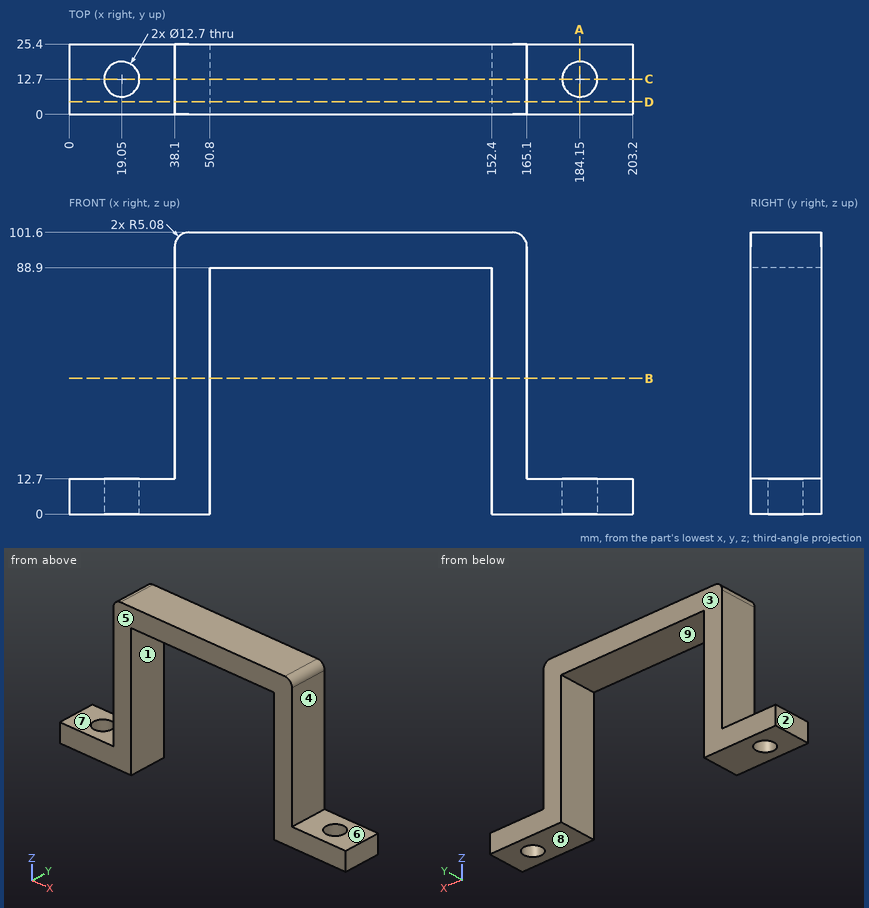
Geometry: see drawing. Coordinates: mm, zero at the bounding-box minimum. A direction names the side the tool comes from. Coordinates: 2 decimals unless noted, no trailing zeros. Order: outer loops, then holes, each group sorted by start corner. A loop starts at its lowest first (then second) coordinate and runs counter-clockwise, first axis right, second up. Notation, with made-up numbers: (-27.5, 40) -> (14.5, 40) arc R10 cw to (14.5, 55) -> close; hole circle Ø9 at (81.25, -12.75). An arc over 180 degrees is marked (long way). Write each question's results on one line, items separated by ' | '. Start each with the question number.
1) Cut plane A-A, the plane x = 184.15. Output: boundary loops of the cut face in (y, z), and give its area (3 significant figures).
2) Material intervals for line 1 along X through (y, z) = (8, 68); line 2 along Y through (x, z) = (19, 5); line 3 along Z through (x, y) = (85.5, 11.25), sorted ascending.
3) Cut plane B-B, the plane z = 49. Output: boundary loops of the cut face in (x, y).
4) Cut plane C-C, the plane y = 12.7. Output: boundary loops of the cut face in (x, z), and give its area (3 significant figures).
5) Set-up query: the marked faces 5, 6, 7, 8 and 9. Return all of +Z, -Z, +X, -X, +Y, -Y with unobstructed straight access to the full face (end or side cutting, diameter ignored); none if empty.
6) Cut plane D-D, the plane y = 4.5. Output: boundary loops of the cut face in (x, z).
7) Mould query, pull axis X, two halves, no side actions, for the marked faces 1, 2, 3 and 4. Classes: released by +X, released by -X, zero draft, split by the parting line, or undercut.
8) First-contact query: pin 1 (14.5 mm diameter, centred on x = 184.15, y = 12.7, fed in from +Z); pin 2 (5 mm diameter, centred on x = 142, y = 4.5, fed in from -Z); pin 3 (2 mm diameter, centred on y = 18.5, z = 77.5, fed in from +X). Flat tips, straight axial feed; report the tip coordinate or a pass-through.
Checks:
1) outline: (0, 0) -> (6.35, 0) -> (6.35, 12.7) -> (0, 12.7) -> close; (19.05, 0) -> (25.4, 0) -> (25.4, 12.7) -> (19.05, 12.7) -> close | area: 161 mm^2
2) line 1: 38.1 to 50.8, 152.4 to 165.1 | line 2: 0 to 6.35, 19.05 to 25.4 | line 3: 88.9 to 101.6
3) outline: (38.1, 0) -> (50.8, 0) -> (50.8, 25.4) -> (38.1, 25.4) -> close; (152.4, 0) -> (165.1, 0) -> (165.1, 25.4) -> (152.4, 25.4) -> close
4) outline: (0, 0) -> (12.7, 0) -> (12.7, 12.7) -> (0, 12.7) -> close; (25.4, 0) -> (50.8, 0) -> (50.8, 88.9) -> (152.4, 88.9) -> (152.4, 0) -> (177.8, 0) -> (177.8, 12.7) -> (165.1, 12.7) -> (165.1, 96.52) arc R5.08 ccw to (160.02, 101.6) -> (43.18, 101.6) arc R5.08 ccw to (38.1, 96.52) -> (38.1, 12.7) -> (25.4, 12.7) -> close; (190.5, 0) -> (203.2, 0) -> (203.2, 12.7) -> (190.5, 12.7) -> close | area: 4,510 mm^2
5) face 5: +Z, -Z, +X, -X, -Y | face 6: +Z, +X, +Y, -Y | face 7: +Z, -X, +Y, -Y | face 8: -Z, +X, -X, +Y, -Y | face 9: -Z, +Y, -Y
6) outline: (0, 0) -> (50.8, 0) -> (50.8, 88.9) -> (152.4, 88.9) -> (152.4, 0) -> (203.2, 0) -> (203.2, 12.7) -> (165.1, 12.7) -> (165.1, 96.52) arc R5.08 ccw to (160.02, 101.6) -> (43.18, 101.6) arc R5.08 ccw to (38.1, 96.52) -> (38.1, 12.7) -> (0, 12.7) -> close
7) face 1: undercut | face 2: released by -X | face 3: zero draft | face 4: released by +X
8) pin 1: z = 12.7 | pin 2: z = 88.9 | pin 3: x = 165.1
